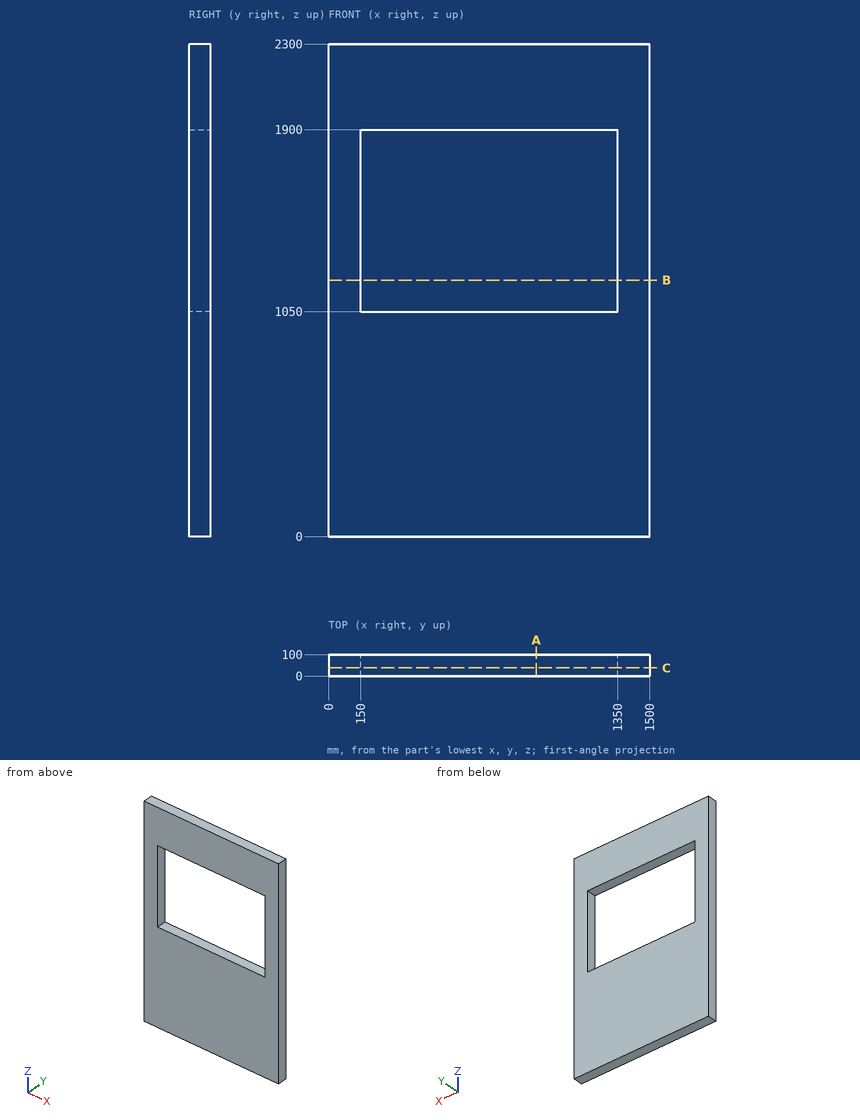
Geometry check sheet. Reference: drawing and pictorial views, mm from the part's lowest x, y, z. Give positions to 0.01 mm unless a question says otherwise; leave off trailing zeros. Loops run counter-clockwise (first coordinate to the right, second up) from the corner with the lowest first, then second, coordinate; pieces in that order, holes last.
1. Section check A-A, the plane x = 970.5. Enter the section's corners in (y, z), then the cut area to 3 significant figures.
2. Section check C-C, the plane y = 38.5. Enter the section's corners in (x, z).
3. Section check B-B, the plane z = 1198. Enter the section's corners in (x, y), then the cut area to 3 significant figures.
4. Thickness scan on line 1 (Z direction, x = 661.5, y = 65); line 2 (X direction, y = 34, z = 1316). Record the ranges inside material, lowest first.
Geometry says:
1. outline: (0, 0) - (100, 0) - (100, 1050) - (0, 1050) - close; (0, 1900) - (100, 1900) - (100, 2300) - (0, 2300) - close
1. area: 145,000 mm2
2. outline: (0, 0) - (1500, 0) - (1500, 2300) - (0, 2300) - close; hole (150, 1050) - (1350, 1050) - (1350, 1900) - (150, 1900) - close
3. outline: (0, 0) - (150, 0) - (150, 100) - (0, 100) - close; (1350, 0) - (1500, 0) - (1500, 100) - (1350, 100) - close
3. area: 30,000 mm2
4. line 1: z = 0 to 1050, 1900 to 2300
4. line 2: x = 0 to 150, 1350 to 1500
